Geometry check sheet. Reference: the model listing, model coordinates, mm. A direction names the side the tool comes from. Round coordinates to 2 decimals unless told otherwise and drop trailing zeros. Write each loop counter-clockwise with the first axis right and the second up, starting at its lowest first coordinate (ties: lowest second). Pieces come first, ordered by that corner, then holes. Notation, with made-up numbers: M 57,-5 L 98,-5 A7 ccw 98,8 Z; hole C 9.5,66.5 d6. An arc over 180 degrees is marked long. Put each result on its own line as item: value. Start each with the question number.
(1) Tool access check on faces 4 (the cylindrical face through (10.07, 10.07, -3.45)), 5 (the flat face through (-15, 20, -6)), 6 (the flat face through (-19, 20, -20)). Record the directions out of +Z, -Z, +X, -X, +Y, -Y that give a thin tool (end or side, any length) a straight path to the whole face; none if there is none.
(2) Section check B-B on y = 30. Count the separate pieces of the cut face and the enclosed holes in it, then the cut area to 3 significant figures.
(3) Mould release check, pull along X, two halves, no side actions. Record for faces 1 (the flat face through (-5, 20, 0)), 2 (the flat face through (-12, 20, -12.5)), 3 (the cylindrical face through (42.77, 20.28, -30.473)): pulls with the +X half, pulls with the -X half, needs draft (parallel to the pull), parting line crosses it, or undercut.
(4) Section check A-A on z = -9. Record the cut outline in (x, y).
(5) Material ranges on probe 1 along Y at (x, z) = (9, -5); probe 2 along X at (y, z) = (24, -7.5); probe 3 along Z at (x, y) = (-14, 18), recorded low to high.
(6) Section check C-C on y = 17. Record the cut outline in (x, z), then the cut area to 3 significant figures.
(7) Gauge pin test, flat ends, axial feed: pin 1 (3.5 mm diameter, centred on y = 10, z = -5, fed in from +X); pin 2 (2.5 mm diameter, centred on x = 3, y = 20, fed in from +Z); pin 3 (8 mm diameter, centred on x = -11.5, y = 8, fed in from -Z). Record the tip position at first contact, or that the pin passes through.
Autodesk Inventor part; units mm, degrees
ref_plane "YZ Plane" through (0, 0, 0) normal (1, 0, 0) x (0, 1, 0)
ref_plane "XZ Plane" through (0, 0, 0) normal (0, 1, 0) x (-1, 0, 0)
ref_plane "XY Plane" through (0, 0, 0) normal (0, 0, 1) x (1, 0, 0)
sketch "スケッチ3" plane through (0, 0, 0) normal (0, 1, 0) x (-1, 0, 0)
  line L0 (0, 0) -> (25, 0)
  line L1 (25, 0) -> (25, -12.5)
  line L2 (25, -12.5) -> (0, -12.5)
  line L3 (0, -12.5) -> (0, 0)
  line L4 (15, 0) -> (10, 0)
  line L5 (10, 0) -> (10, -12.5)
  line L6 (10, -12.5) -> (15, -12.5)
  line L7 (15, -12.5) -> (15, 0)
  dimension "d112" = 25
  dimension "d113" = 12.5
  dimension "d114" = 5
  dimension "d115" = 10
extrude "押し出し1" add sketch "スケッチ3" along normal blind 40 contours L0 L5 L2 L3 | L0 L1 L2 L7
sketch "スケッチ4" plane through (0, 0, 0) normal (1, 0, 0) x (0, 0, -1)
  line L0 (12.5, 0) -> (0, 0)
  line L1 (5, 0) -> (5, 40)
  line L2 (0, 40) -> (12.5, 40)
  line L3 (12.5, 0) -> (12.5, 40)
  line L4 (0, 0) -> (0, 40)
  line L5 (0, 20) -> (12.5, 20)
  point P0 (5, 30)
  point P1 (5, 10)
  dimension "d118" = 7.5
  dimension "d119" = 20
  dimension "d120" = 20
hole "穴1" at (0, 30, -5) at (0, 10, -5) direction (-1, 0, 0) diameter 3.1 end through all
sketch "スケッチ5" plane through (0, 0, 0) normal (0, -1, 0) x (1, 0, 0)
  line L0 (0, -12.5) -> (-10, -12.5)
  line L1 (0, -12.5) -> (-25, -12.5)
  line L2 (-25, -12.5) -> (-25, -17.5)
  line L3 (-25, -17.5) -> (0, -17.5)
  line L4 (0, -17.5) -> (0, -12.5)
  point P0 (0, 0)
  dimension "d128" = 5
extrude "押し出し2" add sketch "スケッチ5" against normal blind 40
sketch "スケッチ6" plane through (0, 0, 0) normal (0, -1, 0) x (1, 0, 0)
  line L0 (-15, -12.5) -> (-10, -12.5)
  line L1 (-12.5, -12.5) -> (-12.5, -232.0211)
  circle A0 centre (-12.5, -142.5) radius 122.5
  line L2 (-25, -17.5) -> (0, -17.5)
  circle A1 centre (-12.5, -142.5) radius 135
  line L3 (0, 0) -> (0, -17.5)
  line L4 (0, -17.5) -> (5, -17.5)
  line L5 (5, -17.5) -> (5, -12.5)
  line L6 (5, -12.5) -> (0, -12.5)
  line L7 (0, -12.5) -> (0, -17.5)
  line L8 (5, -17.5) -> (15, -17.5)
  line L9 (15, -17.5) -> (15, 0)
  line L10 (15, 0) -> (5, 0)
  line L11 (5, 0) -> (5, -17.5)
  line L12 (45, -20.3577) -> (45, -34.3335)
  line L13 (-12.5, -20) -> (-25, -20)
  line L14 (-25, 0) -> (-25, -17.5)
  line L15 (-25, -20) -> (-25, -17.5)
  point P0 (0, -12.5)
  point P1 (-12.5, -17.5)
  point P2 (15, -10.3306)
  point P3 (0, -8.0799)
  point P4 (5, -8.6391)
  dimension "d132" = 270
  dimension "d131" = 245
  dimension "d133" = 5
  dimension "d134" = 5
  dimension "d135" = 10
  dimension "d136" = 17.5
  dimension "d139" = 30
  dimension "d144" = 125
extrude "押し出し3" add sketch "スケッチ6" against normal blind 40 contours L3 L6 L5 L4 | L5 L11 A1 L9 L8 | A1 L11 L10 L9
extrude "押し出し4" add sketch "スケッチ6" against normal blind 40 contours L2 L4 L8 L9 A1 L12 A0 L1 | L1 L13 L15 L2
sketch "スケッチ7" plane through (15, 0, 0) normal (1, 0, 0) x (0, 0, -1)
  circle A0 centre (5, 30) radius 1.55
  circle A1 centre (5, 10) radius 1.55
  point P0 (0, 0)
extrude "押し出し5" cut sketch "スケッチ7" against normal blind 40
fillet "フィレット1" radius 5 1 edges at (45, 20, -34.3335)
fillet "フィレット2" radius 5 1 edges at (45, 20, -20.3577)
properties part number "hand2_14" material "ABS プラスチック"
Answers follow:
1. face 4: +X, -X
1. face 5: +Z, +Y, -Y
1. face 6: -Z, -X, +Y, -Y
2. separate pieces: 4
2. enclosed holes: 0
2. area: 993 mm^2
3. face 1: needs draft
3. face 2: undercut
3. face 3: parting line crosses it
4. outline: M -25,0 L -15,0 L -15,40 L -25,40 Z; M -10,0 L 0,0 L 0,40 L -10,40 Z; M 5,0 L 15,0 L 15,40 L 5,40 Z
5. probe 1: y = 0 to 8.45, 11.55 to 28.45, 31.55 to 40
5. probe 2: x = -25 to -15, -10 to 0, 5 to 15
5. probe 3: z = -20 to -12.5
6. outline: M -25,-20 L -12.5,-20 A122.5 cw 37.94,-30.87 A5 ccw 45,-26.31 L 45,-23.57 A5 ccw 42.02,-19 A135 ccw 15,-10.33 L 15,0 L 5,0 L 5,-12.5 L 0,-12.5 L 0,0 L -10,0 L -10,-12.5 L -15,-12.5 L -15,0 L -25,0 Z
6. area: 1,090 mm^2
7. pin 1: stops at x = 15
7. pin 2: stops at z = -12.5
7. pin 3: stops at z = -20.1
